Build history of the part. All positions in model axes, mm. A direction names the side the tool comes from. Round coordinates to 2 decimals unless told otherwise and drop trailing zeros. Write each loop counter-clockwise with the first axis right and the second up, starting at its lowest first coordinate (ties: lowest second). Pieces come first, ordered by that corner, then holes. Notation, with made-up numbers: (46, 61.25) - (99, 61.25) arc R17 ccw to (99, 89.25) - close; hole circle Ø6 at (-39, -17). An arc over 180 degrees is marked (long way). Write each question's results on one line, items separated by ' | '.
from build123d import *

# Parameters (mm, degrees)
SKETCH1_R           = 6.75
BOSS_EXTRUDE1_DEPTH = 3.175
SKETCH4_R           = 1.27
BOSS_EXTRUDE2_DEPTH = 8.89
CHAMFER1_SIZE       = 5.71
CUT_EXTRUDE1_DEPTH  = 2.54


with BuildPart() as part:
    # Sketch1 → Boss-Extrude1 (new, symmetric)
    with BuildSketch(Plane.XY):
        with BuildLine():
            Line((-9.75, 0), (-9.75, 45))
            Line((-9.75, 45), (9.75, 45))
            Line((9.75, 45), (9.75, 0))
            ThreePointArc((9.75, 0), (0, -9.75), (-9.75, 0))
        make_face()
        Circle(SKETCH1_R, mode=Mode.SUBTRACT)
    extrude(amount=BOSS_EXTRUDE1_DEPTH, both=True)

    # Sketch4 → Boss-Extrude2 (add, symmetric)
    with BuildSketch(Plane.XY):
        with BuildLine():
            Line((-12.7, 57.7), (-9.75, 45))
            Line((-9.75, 45), (9.75, 45))
            Line((9.75, 45), (12.7, 57.7))
            ThreePointArc((12.7, 57.7), (0, 70.4), (-12.7, 57.7))
        make_face()
        with Locations(Location((0, 65.32, 0), (0, 0, 180))):
            Circle(SKETCH4_R, mode=Mode.SUBTRACT)
        with Locations(Location((7.62, 57.7, 0), (0, 0, 180))):
            Circle(SKETCH4_R, mode=Mode.SUBTRACT)
        with Locations(Location((0, 50.08, 0), (0, 0, 180))):
            Circle(SKETCH4_R, mode=Mode.SUBTRACT)
        with Locations(Location((-7.62, 57.7, 0), (0, 0, 180))):
            Circle(SKETCH4_R, mode=Mode.SUBTRACT)
    extrude(amount=BOSS_EXTRUDE2_DEPTH, both=True)

    # Chamfer1
    # the kernel refuses this chamfer: 5.71 mm, written as the material it adds along each edge
    with BuildSketch(Plane(origin=(-9.75, 45, 3.175), x_dir=(0, 0.02749587661058595, 0.9996219169112968), z_dir=(1, 0, 0))) as chamfer1_piece_1_section:
        Polygon((CHAMFER1_SIZE * 0.999621916911, CHAMFER1_SIZE * 0.0274958766106), (-CHAMFER1_SIZE * 0.0274958766106, CHAMFER1_SIZE * 0.999621916911), (0, 0), align=None)
    chamfer1_piece_1 = extrude(amount=19.5, mode=Mode.PRIVATE)
    chamfer1_piece_1 = split(chamfer1_piece_1, bisect_by=Plane(origin=(-9.076297476, 42.099653541, 4.47568677), z_dir=(-0.9740670228457147, -0.2262596627869977, 0)), keep=Keep.TOP, mode=Mode.PRIVATE)
    add(chamfer1_piece_1)
    with BuildSketch(Plane(origin=(-9.75, 45, 3.175), x_dir=(0, 0.02749587661058595, 0.9996219169112968), z_dir=(1, 0, 0))) as chamfer1_piece_2_section:
        Polygon((CHAMFER1_SIZE * 0.999621916911, CHAMFER1_SIZE * 0.0274958766106), (-CHAMFER1_SIZE * 0.0274958766106, CHAMFER1_SIZE * 0.999621916911), (0, 0), align=None)
    chamfer1_piece_2 = extrude(amount=19.5, mode=Mode.PRIVATE)
    chamfer1_piece_2 = split(chamfer1_piece_2, bisect_by=Plane(origin=(-8.84718109, 41.113288082, 5.085534979), z_dir=(0.9740670228457147, 0.2262596627869977, 0)), keep=Keep.TOP, mode=Mode.PRIVATE)
    chamfer1_piece_2 = split(chamfer1_piece_2, bisect_by=Plane(origin=(8.84718109, 41.113288082, 5.085534979), z_dir=(-0.9740670228457147, 0.2262596627869977, 0)), keep=Keep.TOP, mode=Mode.PRIVATE)
    add(chamfer1_piece_2)
    with BuildSketch(Plane(origin=(-9.75, 45, 3.175), x_dir=(0, 0.02749587661058595, 0.9996219169112968), z_dir=(1, 0, 0))) as chamfer1_piece_3_section:
        Polygon((CHAMFER1_SIZE * 0.999621916911, CHAMFER1_SIZE * 0.0274958766106), (-CHAMFER1_SIZE * 0.0274958766106, CHAMFER1_SIZE * 0.999621916911), (0, 0), align=None)
    chamfer1_piece_3 = extrude(amount=19.5, mode=Mode.PRIVATE)
    chamfer1_piece_3 = split(chamfer1_piece_3, bisect_by=Plane(origin=(9.076297476, 42.099653541, 4.47568677), z_dir=(0.9740670228457147, -0.2262596627869977, 0)), keep=Keep.TOP, mode=Mode.PRIVATE)
    add(chamfer1_piece_3)
    with BuildSketch(Plane(origin=(-9.75, 45, -3.175), x_dir=(0, 0.02749587661058595, -0.9996219169112968), z_dir=(1, 0, 0))) as chamfer1_piece_4_section:
        Polygon((CHAMFER1_SIZE * 0.999621916911, -CHAMFER1_SIZE * 0.0274958766106), (-CHAMFER1_SIZE * 0.0274958766106, -CHAMFER1_SIZE * 0.999621916911), (0, 0), align=None)
    chamfer1_piece_4 = extrude(amount=19.5, mode=Mode.PRIVATE)
    chamfer1_piece_4 = split(chamfer1_piece_4, bisect_by=Plane(origin=(-9.076297476, 42.099653541, -4.47568677), z_dir=(-0.9740670228457147, -0.2262596627869977, 0)), keep=Keep.TOP, mode=Mode.PRIVATE)
    add(chamfer1_piece_4)
    with BuildSketch(Plane(origin=(-9.75, 45, -3.175), x_dir=(0, 0.02749587661058595, -0.9996219169112968), z_dir=(1, 0, 0))) as chamfer1_piece_5_section:
        Polygon((CHAMFER1_SIZE * 0.999621916911, -CHAMFER1_SIZE * 0.0274958766106), (-CHAMFER1_SIZE * 0.0274958766106, -CHAMFER1_SIZE * 0.999621916911), (0, 0), align=None)
    chamfer1_piece_5 = extrude(amount=19.5, mode=Mode.PRIVATE)
    chamfer1_piece_5 = split(chamfer1_piece_5, bisect_by=Plane(origin=(-8.84718109, 41.113288082, -5.085534979), z_dir=(0.9740670228457147, 0.2262596627869977, 0)), keep=Keep.TOP, mode=Mode.PRIVATE)
    chamfer1_piece_5 = split(chamfer1_piece_5, bisect_by=Plane(origin=(8.84718109, 41.113288082, -5.085534979), z_dir=(-0.9740670228457147, 0.2262596627869977, 0)), keep=Keep.TOP, mode=Mode.PRIVATE)
    add(chamfer1_piece_5)
    with BuildSketch(Plane(origin=(-9.75, 45, -3.175), x_dir=(0, 0.02749587661058595, -0.9996219169112968), z_dir=(1, 0, 0))) as chamfer1_piece_6_section:
        Polygon((CHAMFER1_SIZE * 0.999621916911, -CHAMFER1_SIZE * 0.0274958766106), (-CHAMFER1_SIZE * 0.0274958766106, -CHAMFER1_SIZE * 0.999621916911), (0, 0), align=None)
    chamfer1_piece_6 = extrude(amount=19.5, mode=Mode.PRIVATE)
    chamfer1_piece_6 = split(chamfer1_piece_6, bisect_by=Plane(origin=(9.076297476, 42.099653541, -4.47568677), z_dir=(0.9740670228457147, -0.2262596627869977, 0)), keep=Keep.TOP, mode=Mode.PRIVATE)
    add(chamfer1_piece_6)

    # Sketch5 → Cut-Extrude1 (cut, symmetric)
    with BuildSketch(Plane.XY):
        with BuildLine():
            Line((-12.7, 57.7), (-9.75, 45))
            Line((-9.75, 45), (9.75, 45))
            Line((9.75, 45), (12.7, 57.7))
            ThreePointArc((12.7, 57.7), (0, 70.4), (-12.7, 57.7))
        make_face()
    extrude(amount=CUT_EXTRUDE1_DEPTH, both=True, mode=Mode.SUBTRACT)


solid = part.part
(1) Two-plate mould, pull along Y, no slides. Class faces 5 (the cylindrical face through (0.17, 48.82, -5.76)), 6 (the cylindrical face through (-7.34, 58.94, -5.76)), 7 (the flat face through (11.246, 51.439, 5.759)), 8 (the flat face through (0, 58, 8.89)): released by +Y, released by -Y, zero draft, split by the parting line, or undercut.
Worked answers:
face 5: undercut | face 6: undercut | face 7: released by -Y | face 8: zero draft
(2) Flat gauge pins, fed straight in: pin 1 Ø9 at (y, z) = (30.5, -0.5) entering from -X; pin 2 Ø10 at (x, y) = (-2.5, 26) entering from +Z (3 decimals); pin 3 Ø5 at (y, z) = (43.5, 1) entering from -X. Where does each tip first touch, or does it go through?
Worked answers:
pin 1: stops at x = -9.75 | pin 2: stops at z = 3.175 | pin 3: stops at x = -9.86
(3) Slice it at A-A, the plane x = 0. State how many separate pieces and enclosed holes the cut face has, and give its area (3 significant figures).
Worked answers:
separate pieces: 6 | enclosed holes: 0 | area: 553 mm2
(4) Slice it at C-C, the plane y = -4. Write the cut outline in (x, z) (3 decimals), and give its area (3 significant figures).
Worked answers:
outline: (-8.892, -3.175) - (-5.437, -3.175) - (-5.437, 3.175) - (-8.892, 3.175) - close; (5.437, -3.175) - (8.892, -3.175) - (8.892, 3.175) - (5.437, 3.175) - close | area: 43.9 mm2
(5) Slice it at D-D, the plane x = 10.5. Write the cut outline in (y, z).
Worked answers:
outline: (48.23, -8.89) - (64.84, -8.89) - (64.84, -2.54) - (48.23, -2.54) - close; (48.23, 2.54) - (64.84, 2.54) - (64.84, 8.89) - (48.23, 8.89) - close
(6) Drill centre lines: probe 1 along X at (y, z) = (57.7, 4.25); probe 2 along Y at (x, z) = (0, 6.5) (3 decimals); probe 3 along Y at (x, z) = (0, 5) (3 decimals). Where is each one in solid material? Low to high. Write a range as [from, to].
Worked answers:
probe 1: x = [-12.7, -8.89], [-6.35, 6.35], [8.89, 12.7] | probe 2: y = [42.615, 48.81], [51.35, 64.05], [66.59, 70.4] | probe 3: y = [41.115, 48.81], [51.35, 64.05], [66.59, 70.4]
(7) Tool access for faces 1 (the flat face through (-9.75, 23, -1)), 2 (the flat face through (0, 58, 2.54)), 3 (the flat face through (9.75, 23, -1)), 4 (the flat face through (0, 21, 3.175)): list every direction of +Z, -Z, +X, -X, +Y, -Y with a clear straight run to the whole face (end or side of a thin tool).
Worked answers:
face 1: +Z, -Z, -X, -Y | face 2: +X, -X, +Y | face 3: +Z, -Z, +X, -Y | face 4: +Z, +X, -X, -Y
(8) Slice it at B-B, the plane y = 50.08. Write the cut outline in (x, z).
Worked answers:
outline: (-10.93, -8.89) - (-1.27, -8.89) - (-1.27, -2.54) - (-10.93, -2.54) - close; (-10.93, 2.54) - (-1.27, 2.54) - (-1.27, 8.89) - (-10.93, 8.89) - close; (1.27, -8.89) - (10.93, -8.89) - (10.93, -2.54) - (1.27, -2.54) - close; (1.27, 2.54) - (10.93, 2.54) - (10.93, 8.89) - (1.27, 8.89) - close
